The listing builds one solid part. Answer for the finished solid, in the listing's coordinates (mm). Give positions to 0.01 mm unless a question says otherwise; leave off trailing zeros. Loops run counter-clockwise (first coordinate to the right, second up) from the corner with the lowest first, then second, coordinate; pieces in that order, holes last.
Item 1: Section B-B, the plane z = 0.8 is taken. Give the vertices of the cut face in (x, y).
Item 2: Section C-C, the plane y = 14.25 is taken. Give the vertices of the cut face in (x, z).
Item 3: Section D-D, the plane x = 0 is taken. Give the vertices of the cut face in (y, z), and give its area (3 significant figures).
Item 4: Section A-A, the plane x = 21 is taken. Give the vertices of the cut face in (y, z).
Item 5: Consider line 1 along Y through (x, z) = (19, 0.9); line 2 along Y through (x, z) = (20.5, 1.8); line 3 along X through (y, z) = (1.5, 1.65). Determine where each line is inside the solid, lowest interval first.
Item 6: Each of these flat-tipped pins is pushed along its axis until it touches: pin 1 Ø10 at (x, y) = (16.5, 10.5) entering from +Z; pin 2 Ø1 at (y, z) = (2.5, 1) entering from +X. Where does it stop, or does it pass through?
from build123d import *

# Parameters (mm, degrees)
SKETCH1_R           = 1
SKETCH1_R_2         = 3
BOSS_EXTRUDE1_DEPTH = 2


with BuildPart() as part:
    # Sketch1 → Boss-Extrude1 (new body)
    with BuildSketch(Plane.XY):
        with BuildLine():
            Line((11.808151179, -0.905709908), (5.779825316, 0.664336707))
            ThreePointArc((5.779825316, 0.664336707), (3.723166432, 0.464621774), (2.283506385, -1.017643645))
            ThreePointArc((2.283506385, -1.017643645), (-0.630092723, -2.419293938), (-2.489805466, 0.225540995))
            ThreePointArc((-2.489805466, 0.225540995), (-3.023512134, 2.221759674), (-4.721460758, 3.399342916))
            Line((-4.721460758, 3.399342916), (-35.248215692, 11.34987999))
            Line((-35.248215692, 11.34987999), (-34.240067334, 15.220750291))
            Line((-34.240067334, 15.220750291), (12.816299536, 2.965160393))
            ThreePointArc((12.816299536, 2.965160393), (14.215899346, 2.938138637), (15.47538955, 3.54911673))
            ThreePointArc((15.47538955, 3.54911673), (24.286630582, -2.088947309), (13.844561325, -2.712585228))
            ThreePointArc((13.844561325, -2.712585228), (13.043119538, -1.564847947), (11.808151179, -0.905709908))
        make_face()
        Circle(SKETCH1_R, mode=Mode.SUBTRACT)
        with Locations((18.964183918, -0.702743317)):
            Circle(SKETCH1_R_2, mode=Mode.SUBTRACT)
    extrude(amount=BOSS_EXTRUDE1_DEPTH)


solid = part.part
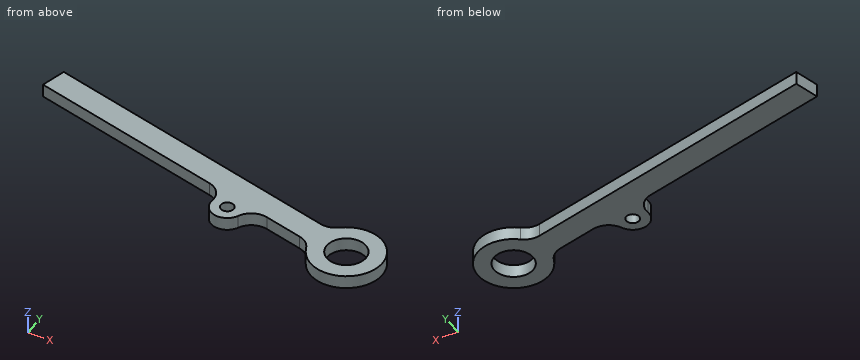
Worked answers:
1. outline: (-35.25, 11.35) - (-4.72, 3.4) arc R3 cw to (-2.49, 0.23) arc R2.5 ccw to (2.28, -1.02) arc R3 cw to (5.78, 0.66) - (11.81, -0.91) arc R3 cw to (13.84, -2.71) arc R5.5 ccw (long way) to (15.48, 3.55) arc R3 cw to (12.82, 2.97) - (-34.24, 15.22) - close; hole circle Ø2 at (0, 0); hole circle Ø6 at (18.96, -0.7)
2. outline: (-34.49, 0) - (-30.51, 0) - (-30.51, 2) - (-34.49, 2) - close
3. outline: (-2.5, 0) - (-1, 0) - (-1, 2) - (-2.5, 2) - close; (1, 0) - (6.3, 0) - (6.3, 2) - (1, 2) - close
3. area: 13.6 mm2
4. outline: (-5.81, 0) - (-2.91, 0) - (-2.91, 2) - (-5.81, 2) - close; (1.5, 0) - (4.41, 0) - (4.41, 2) - (1.5, 2) - close
5. line 1: y = -6.2 to -3.7, 2.3 to 4.8
5. line 2: y = -5.98 to -3.28, 1.87 to 4.58
5. line 3: x = -2.65 to 16.93, 21 to 24
6. pin 1: passes through
6. pin 2: stops at x = 23.75
